Design review of the part shown in the three views and the two pictorial views. Dimensions are in mm from the part's minimum x, y and z. A direction names the side the tool comes from. Round coordinates to 2 decimals unless told otherwise and drop trailing zeros. Loops run counter-clockwise (first coordinate to the right, second up) from the corner with the lowest first, then second, coordinate; pieces in that order, holes last.
1) Take a section at A-A (y = 10). State the section outline as (x, z) points.
2) Insertion check: pin 1 (2 mm diameter, centred on x = 4.5, y = 9, fed in from +Z); pin 2 (5 mm diameter, centred on y = 3.5, z = 5.5, fed in from -X); pin 3 (3 mm diameter, centred on x = 10, y = 10, fed in from +Z); pin 4 (3 mm diameter, centred on y = 8.5, z = 8, fed in from +X). Each pin has a flat end and moves straight along its axis. Give the tip position at first contact, or say it passes through.
3) Take a section at D-D (x = 5.75). State the section outline as (y, z) points.
4) Wall thickness on L1, parallel to Y at x = 10, z = 8.75; L2, parallel to Z at x = 13.5, y = 18.25; L3, parallel to Y at x = 8.5, z = 6.75: over which ranges is each line inside the solid? List them lowest first.
5) Take a section at C-C (z = 10.75). State the section outline as (x, y) points, then the cut area to 3 significant figures.
6) Mouldability with a two-part tool opening along Y and no side actions: class the marked faces 1, 2 and 3 as pulls with the +Y half, pulls with the -Y half, needs draft (parallel to the pull), parting line crosses it, or undercut.
7) Tool access review of the marked faces 4 and 5: name each direction out of +Z, -Z, +X, -X, +Y, -Y from which nothing blocks a thin tool from reaching the whole face with its end or side.
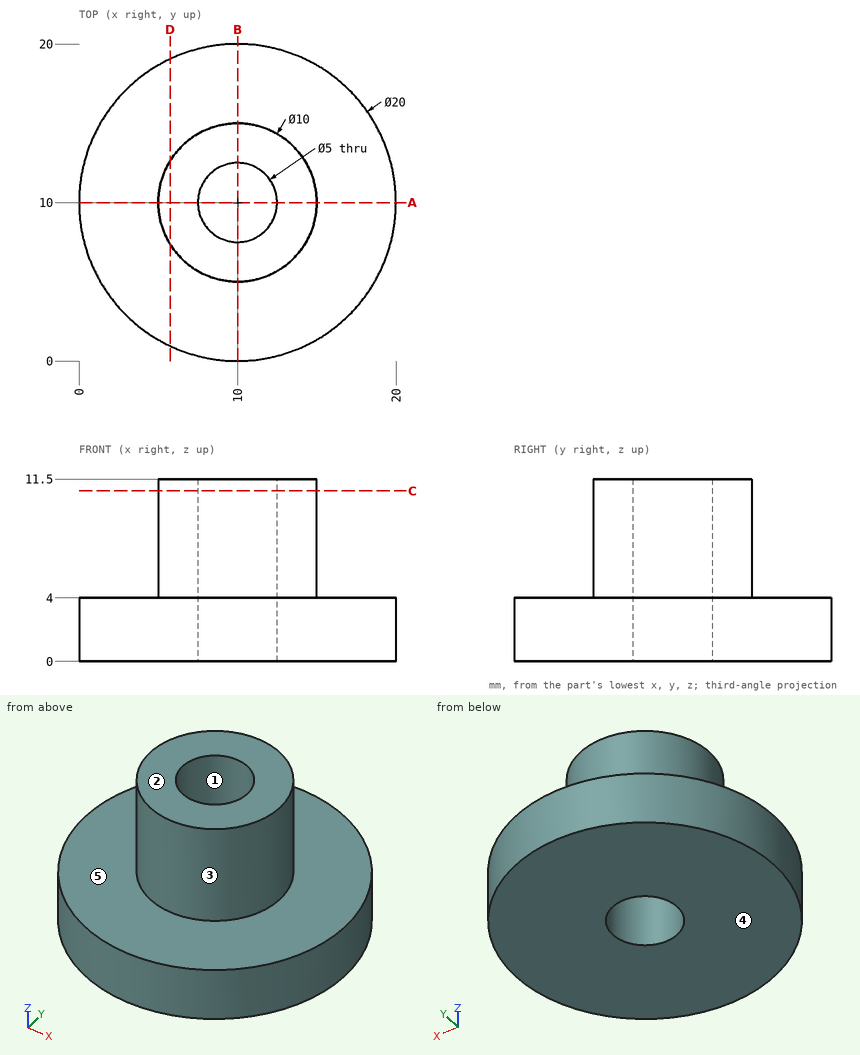
Response:
1. outline: (0, 0) - (7.5, 0) - (7.5, 11.5) - (5, 11.5) - (5, 4) - (0, 4) - close; (12.5, 0) - (20, 0) - (20, 4) - (15, 4) - (15, 11.5) - (12.5, 11.5) - close
2. pin 1: stops at z = 11.5
2. pin 2: stops at x = 1.07
2. pin 3: passes through
2. pin 4: stops at x = 15
3. outline: (0.95, 0) - (19.05, 0) - (19.05, 4) - (12.63, 4) - (12.63, 11.5) - (7.37, 11.5) - (7.37, 4) - (0.95, 4) - close
4. L1: y = 5 to 7.5, 12.5 to 15
4. L2: z = 0 to 4
4. L3: y = 5.23 to 8, 12 to 14.77
5. outline: circle Ø10 at (10, 10); hole circle Ø5 at (10, 10)
5. area: 58.9 mm2
6. face 1: undercut
6. face 2: needs draft
6. face 3: parting line crosses it
7. face 4: -Z, +X, -X, +Y, -Y
7. face 5: +Z
